Autodesk Inventor part; units mm, degrees
ref_plane "YZ Plane" through (0, 0, 0) normal (1, 0, 0) x (0, 1, 0)
ref_plane "XZ Plane" through (0, 0, 0) normal (0, 1, 0) x (-1, 0, 0)
ref_plane "XY Plane" through (0, 0, 0) normal (0, 0, 1) x (1, 0, 0)
sketch "Sketch1" plane through (0, 0, 0) normal (0, 0, 1) x (1, 0, 0)
  line L0 (-54.75, 42.4) -> (54.75, 42.4)
  line L1 (63.55, 42.4) -> (63.55, -42.4)
  line L2 (54.75, -42.4) -> (-54.75, -42.4)
  line L3 (-63.55, -42.4) -> (-63.55, 42.4)
  line L4 (-63.55, 42.4) -> (63.55, -42.4) construction
  line L5 (63.55, 42.4) -> (-63.55, -42.4) construction
  arc A0 (63.55, 42.4) -> (54.75, 42.4) centre (59.15, 42.4) ccw
  line L6 (-63.55, 0) -> (63.55, 0) construction
  line L7 (-8.8, 42.4) -> (-8.8, -42.4) construction
  line L8 (-63.55, 42.4) -> (-54.75, 42.4) construction
  line L9 (-54.75, 42.4) -> (-54.75, 42.4) construction
  arc A1 (-63.55, -42.4) -> (-54.75, -42.4) centre (-59.15, -42.4) ccw
  arc A2 (54.75, -42.4) -> (63.55, -42.4) centre (59.15, -42.4) ccw
  arc A3 (-54.75, 42.4) -> (-63.55, 42.4) centre (-59.15, 42.4) ccw
  point P0 (0, 0)
  dimension "d2" = 127.1
  dimension "d4" = 84.8
  dimension "d10" = 4.4
extrude "Extrusion2" add sketch "Sketch1" along normal blind 5
sketch "Sketch2" plane through (0, 0, 5) normal (0, 0, 1) x (1, 0, 0)
  arc A0 (-63.55, -42.4) -> (-54.75, -42.4) centre (-59.15, -42.4) ccw
  circle A1 centre (-59.15, -42.4) radius 3.5
  point P0 (0, 0)
  dimension "d14" = 7
extrude "Extrusion3" add sketch "Sketch2" along normal blind 10
sketch "Sketch3" plane through (-54.75, -42.4, 0) normal (0, -1, 0) x (1, 0, 0)
  line L0 (0, 5) -> (109.5, 5)
  line L1 (0, 0) -> (0, 5)
  line L2 (54.75, 0) -> (54.75, 1.8) construction
  line L3 (54.75, 1.8) -> (69.75, 1.8)
  line L4 (69.75, 1.8) -> (69.75, 5)
  line L5 (39.75, 5) -> (39.75, 1.8)
  line L6 (39.75, 1.8) -> (54.75, 1.8)
  dimension "d18" = 1.8
  dimension "d19" = 15
extrude "Extrusion4" add sketch "Sketch3" along normal blind 8
ref_plane "Work Plane1" through (-54.75, 0, 0) normal (0, -1, 0) x (1, 0, 0)
mirror "Mirror1" about plane through (-54.75, 0, 0) normal (0, -1, 0) of "Extrusion4"
fillet "Fillet1" radius 1 4 edges at (-15, -50.4, 3.4) (15, -50.4, 3.4) (15, 50.4, 3.4) (-15, 50.4, 3.4)
properties part number "BaseTI stage insert"
Could you check a few things on this model? Use its own coordinates, in mm. A direction names the side the tool comes from. Coordinates: 2 decimals unless noted, no trailing zeros. Loops run counter-clockwise (first coordinate to the right, second up) from the corner with the lowest first, then second, coordinate; pieces in that order, holes last.
1. Imagine slicing it at B-B (y = 14). Please give me the cut outline in (x, z), and give its area (4 significant figures).
2. For P1, Ø1.6, axis at y = -47, z = 3, coming from the +X side; P2, Ø4, axis at x = -2.5, y = 45, coming from the -Z side; P3, Ø3.5, axis at y = 44.5, z = 3, coming from the -X side, each with a flat end and sliding along its axis, tell me the tip position at first contact or that it passes through.
3. I need wall thicknesses on L1, parallel to X at y = 46, z = 3.75; L2, parallel to Z at x = -3, y = -26; L3, parallel to Y at x = 25.5, z = 1.25. Which ranges of each line are inside material? Lowest first, please.
4. Imagine slicing it at C-C (z = 10.5). Please give me the cut outline in (x, y).
5. Imagine slicing it at D-D (x = 59.15). Please give me the cut outline in (y, z), and give its area (3 significant figures).
6. For faces 1 (the face through (15, 46, 3)), 2 (the face through (0, 46, 1.8)), 3 (the face through (-63.55, -1, 2)), 4 (the face through (0, -46, 1.8)), 5 (the face through (15, -46, 3)), which set-ups out of +Z, -Z, +X, -X, +Y, -Y let a thin tool reach every point of the face, with its end or its side?
7. We'd pull the mould along X, two halves only. Please class faces 6 (the face through (-55.81, -43.45, 9.93)), 7 (the face through (-1, 1, 5)), 8 (the face through (59.2, -46.8, 2.5)): released by +X, released by -X, zero draft, split by the parting line, or undercut.
8. Imagine slicing it at A-A (x = -59.15). Please give me the cut outline in (y, z), and give its area (3 significant figures).
Computed values:
1. outline: (-63.55, 0) - (63.55, 0) - (63.55, 5) - (-63.55, 5) - close
1. area: 635.5 mm2
2. P1: stops at x = 61.37
2. P2: stops at z = 1.8
2. P3: stops at x = -63.54
3. L1: x = -61.68 to -56.62, -15 to 15, 56.62 to 61.68
3. L2: z = 0 to 5
3. L3: y = -42.4 to 42.4
4. outline: circle Ø7 at (-59.15, -42.4)
5. outline: (-46.8, 0) - (46.8, 0) - (46.8, 5) - (-46.8, 5) - close
5. area: 468 mm2
6. face 1: +Z, -Z, +Y
6. face 2: -Z, +Y
6. face 3: +Z, -Z, -X, +Y, -Y
6. face 4: -Z, -Y
6. face 5: +Z, -Z, -Y
7. face 6: split by the parting line
7. face 7: zero draft
7. face 8: undercut
8. outline: (-46.8, 0) - (46.8, 0) - (46.8, 5) - (-38.9, 5) - (-38.9, 15) - (-45.9, 15) - (-45.9, 5) - (-46.8, 5) - close
8. area: 538 mm2
